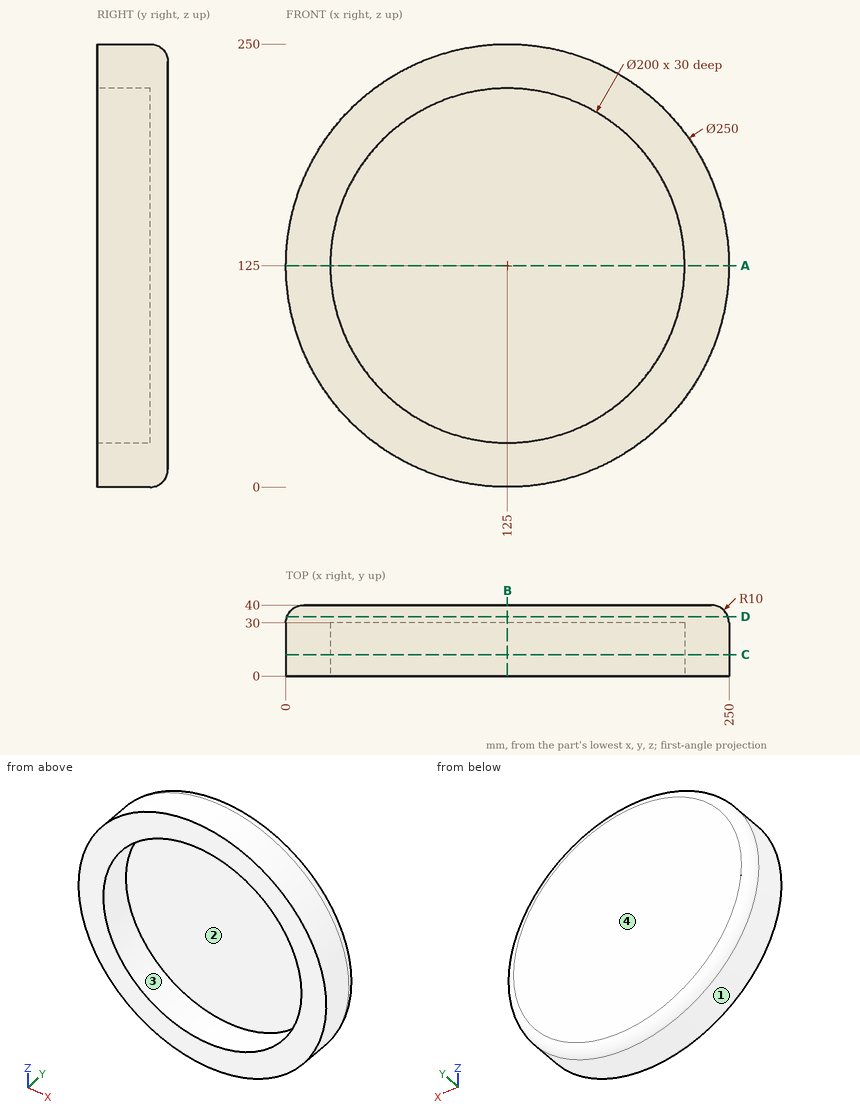
Here's the drawing with two shaded views (mm, measured from the low corner). I have some questions. Coordinates: 2 decimals unless noted, no trailing zeros. Loops run counter-clockwise (first coordinate to the right, second up) from the corner with the lowest first, then second, coordinate; pieces in that order, holes last. Notation, with made-up numbers: (72, 53) - (123, 53) arc R24 cw to (123, 91) - close; hole circle Ø1 at (-14, 26.25). An arc over 180 degrees is marked (long way). Answer as CSV lines item,"result". Start each with the question number.
1) For pin 1 (10 mm diameter, centred on x = 186.5, y = 9.5, fed in from -Z); pin 2 (1 mm diameter, centred on x = 209.5, y = 29, fed in from +Z); pin 3 (1 mm diameter, centred on y = 11, z = 166, fed in from +X), each with a flat end and sliding along its axis, tell me the tip position at first contact or that it passes through.
2) Suppose I cut it at B-B (x = 125). Please give me the cut outline in (y, z), plus the area to 3 significant figures.
3) Suppose I cut it at C-C (y = 12). Please give me the cut outline in (x, z), plus the area to 3 significant figures.
4) Thinking about a two-plate mould opening in X: for the marked faces 1, 2, 3 and 4, which applies, pulls with the +X half, pulls with the -X half, needs draft (parallel to the pull), parting line crosses it, or undercut?
5) Suppose I cut it at D-D (y = 33.5). Please give me the cut outline in (x, z) (1 decimal), plus the area to 3 significant figures.
6) Suppose I cut it at A-A (z = 125). Please give me the cut outline in (x, y), plus the area to 3 significant figures.
7) I need wall thicknesses on line 1 (X direction, y = 22, z = 125); line 2 (Y direction, x = 77, z = 77.5); line 3 (Z direction, x = 80.5, y = 19.5). Which ranges of each line are inside material? Lowest first, please. Write a range as from..to.
Check result:
1,pin 1,"stops at z = 13.5"
1,pin 2,"stops at z = 217.57"
1,pin 3,"stops at x = 243.26"
2,outline,"(0, 0) - (30, 0) arc R10 ccw to (40, 10) - (40, 240) arc R10 ccw to (30, 250) - (0, 250) - (0, 225) - (30, 225) - (30, 25) - (0, 25) - close"
2,area,"3,960 mm²"
3,outline,"circle Ø250 at (125, 125); hole circle Ø200 at (125, 125)"
3,area,"17,700 mm²"
4,face 1,"parting line crosses it"
4,face 2,"undercut"
4,face 3,"undercut"
4,face 4,"needs draft"
5,outline,"circle Ø248.7 at (125, 125)"
5,area,"48,600 mm²"
6,outline,"(0, 0) - (25, 0) - (25, 30) - (225, 30) - (225, 0) - (250, 0) - (250, 30) arc R10 ccw to (240, 40) - (10, 40) arc R10 ccw to (0, 30) - close"
6,area,"3,960 mm²"
7,line 1,"x = 0..25, 225..250"
7,line 2,"y = 30..40"
7,line 3,"z = 8.19..35.45, 214.55..241.81"
